Work out the finished part from the listing and answer in its coordinate system (mm). Face numbers are marked on the shaded views. Coordinates: 2 decimals unless noted, no trailing zeros. Order: outer loops, then holes, each group sorted by start corner. A loop starts at its lowest first (then second) coordinate and runs counter-clockwise, first axis right, second up. Notation, with made-up numbers: (-14, -29) -> (10, -29) arc R30 cw to (10, -1) -> close; hole circle Ø7 at (85, 13). An arc over 180 degrees is marked (long way). Use one line per item in the form item = value.
from build123d import *

# Parameters (mm, degrees)
F0_W     = 15.6
F0_H     = 36.5
F1_DEPTH = 38
F2_T     = -2
F3_R     = 1


with BuildPart() as f1:
    # F0 (on Top) → F1 (new body)
    with BuildSketch(Plane.XY):
        with Locations((7.8, 18.25)):
            Rectangle(F0_W, F0_H)
    extrude(amount=F1_DEPTH)

    # F2
    f2_openings = [f1.faces().sort_by_distance(p)[0] for p in [
        (7.8, 18.25, 38),
    ]]
    offset(amount=F2_T, openings=f2_openings)

    # F3
    f3_edges = [f1.edges().sort_by_distance(p)[0] for p in [
        (15.6, 0, 19),
        (15.6, 36.5, 19),
    ]]
    fillet(f3_edges, radius=F3_R)


solid = f1.part
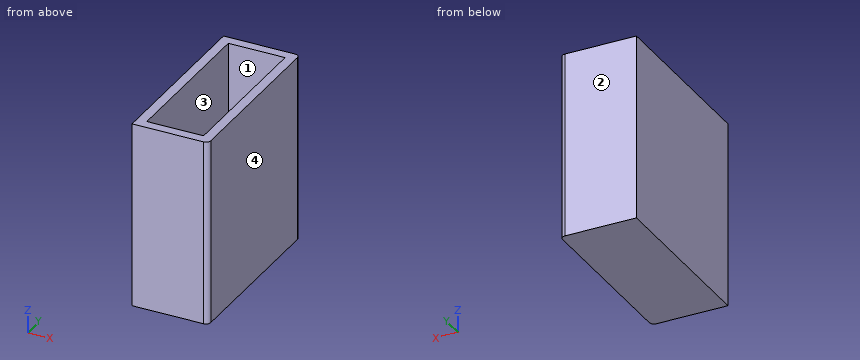
(1) Section B-B on y = 22 is taken. Write down the section's boundary in (x, z).
Data:
outline = (0, 0) -> (15.6, 0) -> (15.6, 38) -> (13.6, 38) -> (13.6, 2) -> (2, 2) -> (2, 38) -> (0, 38) -> close
(2) Straight lines are drawn through the part: line 1 along X through (y, z) = (29, 22); line 2 along Y through (x, z) = (7.5, 15.5); line 3 along Z through (x, y) = (8.25, 30). For each, find the intervals that lie inside material, in ascending order.
Data:
line_1 = 0 to 2, 13.6 to 15.6
line_2 = 0 to 2, 34.5 to 36.5
line_3 = 0 to 2
(3) Each of these flat-tipped pins is pushed along its axis until it touches: P1, Ø4, axis at x = 8, y = 13.5, coming from the +Z side; P2, Ø1.5, axis at y = 8.5, z = 24.5, coming from the -X side. Where does it stop, or does it pass through?
Data:
P1 = 2
P2 = 0
(4) Section C-C on x = 5 is taken. Write down the section's boundary in (y, z), plus the area to 3 significant figures.
Data:
outline = (0, 0) -> (36.5, 0) -> (36.5, 38) -> (34.5, 38) -> (34.5, 2) -> (2, 2) -> (2, 38) -> (0, 38) -> close
area = 217 mm²
(5) The mould has two halves that part along X. Classify the marked faces 1, 2, 3 and 4: released by +X, released by -X, zero draft, split by the parting line, or undercut.
Data:
face_1 = undercut
face_2 = zero draft
face_3 = undercut
face_4 = released by +X
(6) Section A-A on z = 15.5 is taken. Write down the section's boundary in (x, y), plus the area to 3 significant figures.
Data:
outline = (0, 0) -> (14.6, 0) arc R1 ccw to (15.6, 1) -> (15.6, 35.5) arc R1 ccw to (14.6, 36.5) -> (0, 36.5) -> close; hole (2, 2) -> (13.6, 2) -> (13.6, 34.5) -> (2, 34.5) -> close
area = 192 mm²
